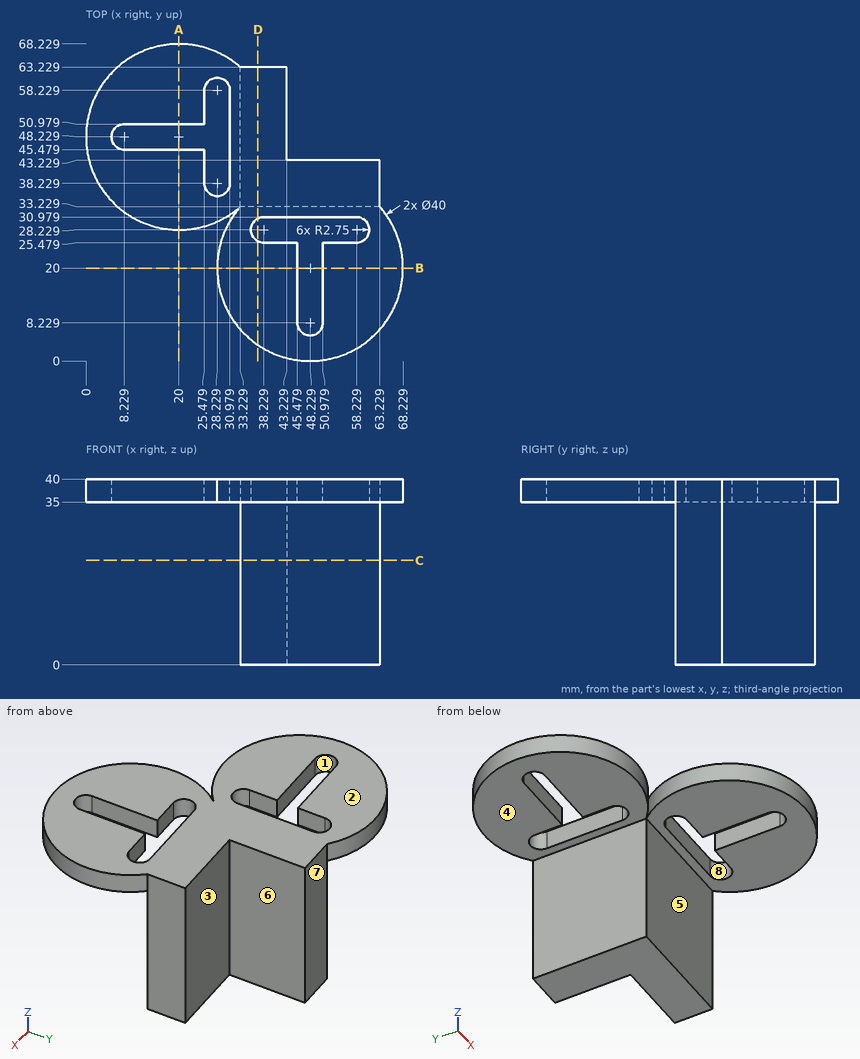
Geometry check sheet. Reference: drawing and pictorial views, mm from the part's lowest x, y, z. A direction names the side the tool comes from. Round coordinates to 2 decimals unless told otherwise and drop trailing zeros. Order: outer loops, then holes, each group sorted by start corner. A loop starts at its lowest first (then second) coordinate and runs counter-clockwise, first axis right, second up. Notation, with made-up numbers: M 29.5,58 L 88.5,58 A19 ccw 88.5,66 Z; hole C 14.25,-17.75 d1. An arc over 180 degrees is marked long. Answer in a Markdown table with one row per item.
(1) Sectioned sample at A-A, the plane x = 20. Record the cut outline in (y, z), and give its area (4 significant figures).
Responses:
| item | result |
|---|---|
| outline | M 28.23,35 L 45.48,35 L 45.48,40 L 28.23,40 Z; M 50.98,35 L 68.23,35 L 68.23,40 L 50.98,40 Z |
| area | 172.5 mm² |
(2) Sectioned sample at C-C, the plane z = 22.5. Record the cut outline in (x, y).
Responses:
| item | result |
|---|---|
| outline | M 33.23,33.23 L 63.23,33.23 L 63.23,43.23 L 43.23,43.23 L 43.23,63.23 L 33.23,63.23 Z |
(3) Tool access check on the marked faces 1, 2, 3, 4 and 5. Record the directions out of +Z, -Z, +X, -X, +Y, -Y that give a thin tool (end or side, any length) a straight path to the whole face; none if there is none.
Responses:
| item | result |
|---|---|
| face 1 | +Z, -Z |
| face 2 | +Z, +X, -X, +Y, -Y |
| face 3 | +Z, -Z, +X, +Y |
| face 4 | -Z, -X, +Y, -Y |
| face 5 | -Z, +X, -X, -Y |
(4) Sectioned sample at D-D, the plane x = 37. Record the cut outline in (y, z).
Responses:
| item | result |
|---|---|
| outline | M 3.45,35 L 25.77,35 L 25.77,40 L 3.45,40 Z; M 30.69,35 L 33.23,35 L 33.23,0 L 63.23,0 L 63.23,40 L 30.69,40 Z |
(5) Scan lines: probe 1 along X at (y, z) = (49, 19.5); probe 2 along Y at (x, z) = (48.5, 38.5). Record each from-to range of solid material in increasing order. Write a range as from..to.
Responses:
| item | result |
|---|---|
| probe 1 | x = 33.23..43.23 |
| probe 2 | y = 0..5.49, 30.98..43.23 |
(6) Draft check along Y on the marked faces 6, 7 and 8. Enter one of: released by +Y, released by -Y, zero draft, split by the parting line, or undercut.
Responses:
| item | result |
|---|---|
| face 6 | zero draft |
| face 7 | released by +Y |
| face 8 | undercut |
(7) Go/stop test with flat-tipped pins: P1, Ø8, axis at x = 37, z = 15.5, coming from the +Y side; P2, Ø6, axis at y = 53, z = 25.5, coming from the +X side; P3, Ø16.5, axis at x = 55, y = 17.5, coming from the -Z side. Record where each tip stops, or that it passes through.
Responses:
| item | result |
|---|---|
| P1 | stops at y = 63.23 |
| P2 | stops at x = 43.23 |
| P3 | stops at z = 35 |
